from build123d import *

# Parameters (mm, degrees)
BOSS_EXTRUDE1_DEPTH = 127
BOSS_EXTRUDE2_DEPTH = 38.1
FILLET1_R           = 1
CUT_EXTRUDE1_DEPTH  = 166.676690047


# Read off the part's stored shape, not the designer's step: Mirror1
with BuildPart() as part:
    # Sketch2 → Boss-Extrude1 (new body)
    with BuildSketch(Plane.XY):
        with BuildLine():
            Line((-71.414284285, -70), (71.414284285, -70))
            ThreePointArc((71.414284285, -70), (0, -100), (-71.414284285, -70))
        make_face()
    extrude(amount=BOSS_EXTRUDE1_DEPTH)

    # Sketch3 → Boss-Extrude2 (add)
    with BuildSketch(Plane(origin=(0, -70, 0), x_dir=(1, 0, 0), z_dir=(0, 1, 0))):
        with BuildLine():
            Line((-52.364284285, -127), (-52.364284285, -117.475))
            ThreePointArc((-52.364284285, -117.475), (-50.504412346, -112.984871939), (-46.014284285, -111.125))
            Line((-46.014284285, -111.125), (-33.314284285, -111.125))
            ThreePointArc((-33.314284285, -111.125), (-28.824156225, -112.984871939), (-26.964284285, -117.475))
            Line((-26.964284285, -117.475), (-26.964284285, -127))
            Line((-26.964284285, -127), (-33.314284285, -127))
            Line((-33.314284285, -127), (-33.314284285, -123.825))
            Line((-33.314284285, -123.825), (-30.139284285, -123.825))
            Line((-30.139284285, -123.825), (-30.139284285, -120.65))
            Line((-30.139284285, -120.65), (-39.664284285, -114.3))
            Line((-39.664284285, -114.3), (-49.189284285, -120.65))
            Line((-49.189284285, -120.65), (-49.189284285, -123.825))
            Line((-49.189284285, -123.825), (-46.014284285, -123.825))
            Line((-46.014284285, -123.825), (-46.014284285, -127))
            Line((-46.014284285, -127), (-52.364284285, -127))
        make_face()
    extrude(amount=BOSS_EXTRUDE2_DEPTH)

    # Fillet1
    fillet1_edges = [part.edges().sort_by_distance(p)[0] for p in [
        (-46.014284285, -50.95, 123.825),
        (-49.189284285, -50.95, 123.825),
        (-49.189284285, -50.95, 120.65),
        (-39.664284285, -50.95, 114.3),
        (-30.139284285, -50.95, 120.65),
        (-30.139284285, -50.95, 123.825),
        (-33.314284285, -50.95, 123.825),
    ]]
    fillet(fillet1_edges, radius=FILLET1_R)

    # Sketch5 → Cut-Extrude1 (cut, symmetric)
    with BuildSketch(Plane(origin=(0, 0, 111.125), x_dir=(-1, 0, 0), z_dir=(0, 0, -1))):
        with BuildLine():
            Line((43.339284285, -38.25), (43.339284285, -63.65))
            ThreePointArc((43.339284285, -63.65), (39.664284285, -67.325), (35.989284285, -63.65))
            Line((35.989284285, -63.65), (35.989284285, -38.25))
            ThreePointArc((35.989284285, -38.25), (39.664284285, -34.575), (43.339284285, -38.25))
        make_face()
    extrude(amount=CUT_EXTRUDE1_DEPTH, both=True, mode=Mode.SUBTRACT)

    # Mirror1: part across plane


with BuildPart() as part_1:
    add(part.part)
    add(part.part.mirror(Plane(origin=(0, 0, 0), x_dir=(0, 0, 1), z_dir=(1, 0, 0))))


solid = part_1.part
CAD build for the part. Positions are in the model's coordinates, mm. A direction names the side the tool comes from. Round coordinates to 2 decimals unless told otherwise and drop trailing zeros. Write each loop counter-clockwise with the first axis right and the second up, starting at its lowest first coordinate (ties: lowest second). Pieces come first, ordered by that corner, then holes. Notation, with made-up numbers: M -14,-37 L 30,-37 A14 cw 30,-32 Z; hole C 59,18 d9. An arc over 180 degrees is marked long. Use a Markdown table: item, result. Add a question column.
1. Pull direction Z, two halves, no side cores. Call faces 1 (the face through (-33.84, -51.217, 118.183)), 2 (the face through (1, -73, 127)), 3 (the face through (-1, -70, 63)): released by +Z, released by -Z, zero draft, split by the parting line, or undercut.
2. Slice it at C-C on y = -80. Give the cut face in (x, z), then the cut area to 3 significant figures.
3. Slice it at B-B on z = 60. Give the cut face in (x, y), then the cut area to 3 significant figures.
4. Drill centre lines: probe 1 along X at (y, z) = (-56, 112); probe 2 along X at (y, z) = (-43.5, 113.5); probe 3 along Z at (x, y) = (-31, -64.5). Where is each one in solid material? Low to high.
5. Slice it at D-D on x = 18. Give the cut face in (y, z), then the cut area to 3 significant figures.
6. 3-axis set-ups, long thin cutter, end or side, ignore diameter. For faces 4 (the face through (-35.5, -51.2, 111.125)), 5 (the face through (45.369, -51.217, 118.103)), 6 (the face through (26.964, -51, 122)): which of +Z, -Z, +X, -X, +Y, -Y reach the whole face in a straight line?
7. Slice it at A-A on y = -48. Give the number of separate pieces and of enclosed holes in the cut face, then the cut area to 3 significant figures.
8. Flat gauge pins, fed straight in: P1, Ø8, axis at x = -48.5, y = -55.5, coming from the -Z side (3 decimals); P2, Ø2, axis at x = -50, z = 68, coming from the -Y side; P3, Ø6, axis at x = -43, z = 123.5, coming from the +Y side; P4, Ø12, axis at x = -31, y = -69.5, coming from the -Z side. Where does each tip first touch, or does it go through?
Reply:
| question | item | result |
|---|---|---|
| 1 | face 1 | undercut |
| 1 | face 2 | released by +Z |
| 1 | face 3 | zero draft |
| 2 | outline | M -60,0 L 60,0 L 60,127 L -60,127 Z |
| 2 | area | 15,200 mm^2 |
| 3 | outline | M -71.41,-70 A100 ccw 71.41,-70 Z |
| 3 | area | 2,950 mm^2 |
| 4 | probe 1 | x = -49.23 to -43.34, -35.99 to -30.1, 30.1 to 35.99, 43.34 to 49.23 |
| 4 | probe 2 | x = -50.97 to -43.34, -35.99 to -28.36, 28.36 to 35.99, 43.34 to 50.97 |
| 4 | probe 3 | z = 111.56 to 120.08, 123.82 to 127 |
| 5 | outline | M -98.37,0 L -70,0 L -70,127 L -98.37,127 Z |
| 5 | area | 3,600 mm^2 |
| 6 | face 4 | -Z, +X, -X, +Y |
| 6 | face 5 | +Y |
| 6 | face 6 | +Z, -Z, +Y |
| 7 | separate pieces | 4 |
| 7 | enclosed holes | 0 |
| 7 | area | 385 mm^2 |
| 8 | P1 | stops at z = 111.125 |
| 8 | P2 | stops at y = -87.17 |
| 8 | P3 | stops at y = -70 |
| 8 | P4 | stops at z = 0 |
